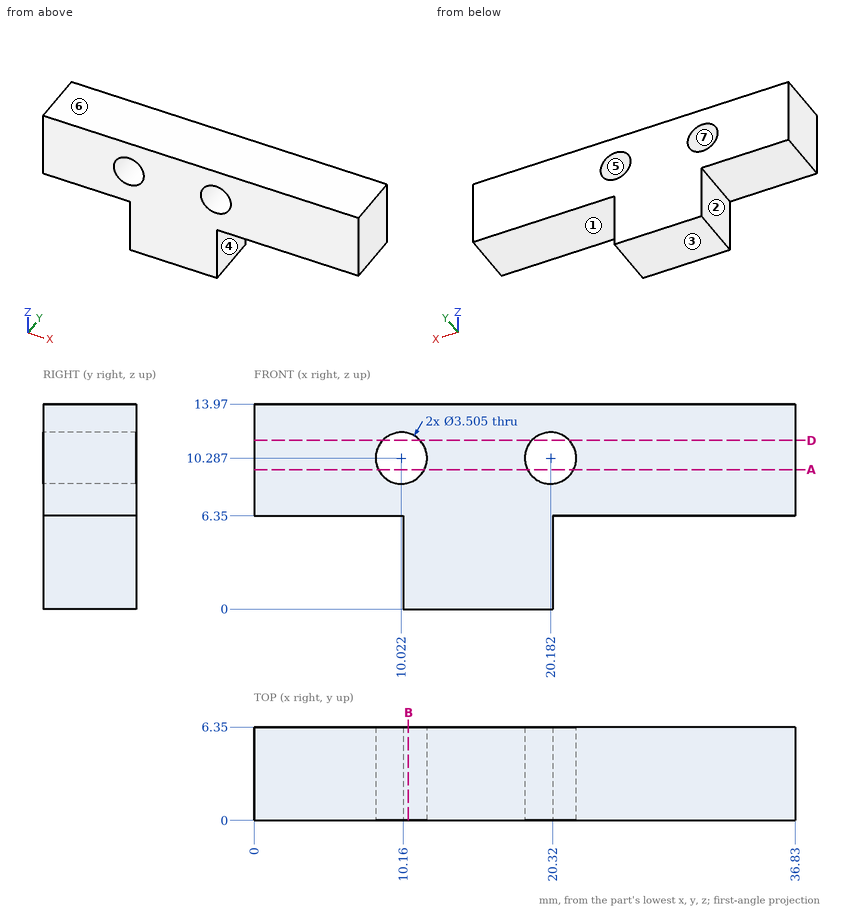
Verification items for this drawing (mm, ordinates from the low corner). A direction names the side the tool comes from. Give positions to 0.01 mm unless a question says otherwise; leave off trailing zeros. Loops run counter-clockwise (first coordinate to the right, second up) from the corner with the lowest first, then second, coordinate; pieces in that order, holes last. Notation, with made-up numbers: M -32,10.5 L -22,10.5 A28 ccw -22,30.5 Z; hole C -13,-11 d1. An arc over 180 degrees is marked long. Write item = value, one per line. Start each with the question number.
1. Section check B-B, the plane x = 10.5. Enter the section's corners in (y, z), plus the area to 3 significant figures.
2. Draft check along Z on the marked faces 4, 5, 6 and 7. Enter one of: +Z half, -Z half, draft (parallel to the pull), parting line (faces both ways), or undercut.
3. Thickness scan on probe 1 along X at (y, z) = (5, 10.25); probe 2 along X at (y, z) = (5.25, 11); probe 3 along Z at (x, y) = (24, 4). Record the ranges inside material, lowest first.
4. Go/stop test with flat-tipped pins: P1, Ø3, axis at y = 2.5, z = 4, coming from the +X side; P2, Ø3, axis at x = 27, y = 4.5, coming from the -Z side. Record where each tip stops, or that it passes through.
5. Tool access check on the marked faces 1, 2 and 3. Record the directions out of +Z, -Z, +X, -X, +Y, -Y that give a thin tool (end or side, any length) a straight path to the whole face; none if there is none.
6. Section check D-D, the plane z = 11.5. Enter the section's corners in (x, y), plus the area to 3 significant figures.
7. Section check A-A, the plane z = 9.5. Give the number of separate pieces and of enclosed holes in the cut face, plus the area to 3 significant figures.
Values follow:
q1.outline = M 0,0 L 6.35,0 L 6.35,8.6 L 0,8.6 Z; M 0,11.97 L 6.35,11.97 L 6.35,13.97 L 0,13.97 Z
q1.area = 67.3 mm^2
q2.face_4 = draft
q2.face_5 = undercut
q2.face_6 = +Z half
q2.face_7 = undercut
q3.probe_1 = 0 to 8.27, 11.77 to 18.43, 21.93 to 36.83
q3.probe_2 = 0 to 8.42, 11.62 to 18.58, 21.78 to 36.83
q3.probe_3 = 6.35 to 13.97
q4.P1 = 20.32
q4.P2 = 6.35
q5.face_1 = -Z, +X, +Y, -Y
q5.face_2 = -Z, -X, +Y, -Y
q5.face_3 = -Z, +X, -X, +Y, -Y
q6.outline = M 0,0 L 8.76,0 L 8.76,6.35 L 0,6.35 Z; M 11.29,0 L 18.92,0 L 18.92,6.35 L 11.29,6.35 Z; M 21.45,0 L 36.83,0 L 36.83,6.35 L 21.45,6.35 Z
q6.area = 202 mm^2
q7.separate_pieces = 3
q7.enclosed_holes = 0
q7.area = 194 mm^2
